Design review of the part built by this model. Coordinates are the model's own, in mm. A direction names the side the tool comes from. Round coordinates to 2 decimals unless told otherwise and drop trailing zeros. Order: outer loops, then holes, each group sorted by start corner. A loop starts at its lowest first (then second) coordinate and runs counter-clockwise, first axis right, second up. Notation, with made-up numbers: M 1.5,26 L 51.5,26 A26 ccw 51.5,48 Z; hole C 47.25,77.5 d5. An arc over 180 degrees is marked long. Write item = value, one per line. Start each with the question number.
```python
from build123d import *

# Parameters (mm, degrees)
SKETCH1_R           = 3.45
BOSS_EXTRUDE1_DEPTH = 2
BOSS_EXTRUDE2_START = 8.75
BOSS_EXTRUDE2_DEPTH = 8.75
CIRPATTERN1_COUNT   = 4


with BuildPart() as part:
    # Sketch1 → Boss-Extrude1 (new body)
    with BuildSketch(Plane(origin=(0, 0, 0), x_dir=(1, 0, 0), z_dir=(0, 1, 0))):
        with BuildLine():
            ThreePointArc((28.363609444, -42.985528487), (38.899494937, -38.899494937), (42.985528487, -28.363609444))
            ThreePointArc((42.985528487, -28.363609444), (51.5, 0), (42.985528487, 28.363609444))
            ThreePointArc((42.985528487, 28.363609444), (38.899494937, 38.899494937), (28.363609444, 42.985528487))
            ThreePointArc((28.363609444, 42.985528487), (0, 51.5), (-28.363609444, 42.985528487))
            ThreePointArc((-28.363609444, 42.985528487), (-38.899494937, 38.899494937), (-42.985528487, 28.363609444))
            ThreePointArc((-42.985528487, 28.363609444), (-51.5, 0), (-42.985528487, -28.363609444))
            ThreePointArc((-42.985528487, -28.363609444), (-38.899494937, -38.899494937), (-28.363609444, -42.985528487))
            ThreePointArc((-28.363609444, -42.985528487), (0, -51.5), (28.363609444, -42.985528487))
        make_face()
        with Locations(Location((14.5, 14.5, 0), (0, 0, 270))):
            Circle(SKETCH1_R, mode=Mode.SUBTRACT)
        with Locations(Location((-14.5, 14.5, 0), (0, 0, 270))):
            Circle(SKETCH1_R, mode=Mode.SUBTRACT)
        with Locations(Location((-14.5, -14.5, 0), (0, 0, 270))):
            Circle(SKETCH1_R, mode=Mode.SUBTRACT)
        with Locations(Location((14.5, -14.5, 0), (0, 0, 270))):
            Circle(SKETCH1_R, mode=Mode.SUBTRACT)
    extrude(amount=BOSS_EXTRUDE1_DEPTH)

    # Sketch2 → Boss-Extrude2 (add)
    with BuildSketch(Plane.XZ.offset(BOSS_EXTRUDE2_START)):
        with BuildLine():
            Line((43.690302721, -24.313729622), (45.001011803, -25.043141511))
            ThreePointArc((45.001011803, -25.043141511), (51.499991825, 0.029017326), (44.972762458, 25.093836632))
            Line((44.972762458, 25.093836632), (43.690302721, 24.313729622))
            ThreePointArc((43.690302721, 24.313729622), (50, 0), (43.690302721, -24.313729622))
        make_face()
    boss_extrude2 = extrude(amount=-BOSS_EXTRUDE2_DEPTH)

    # CirPattern1: Boss-Extrude2 ×4 about axis
    cirpattern1_axis = Axis((0, 0, 0), (0, 1, 0))
    for i in range(1, CIRPATTERN1_COUNT):
        add(boss_extrude2.rotate(cirpattern1_axis, i * 360 / CIRPATTERN1_COUNT))


solid = part.part
```
(1) Consider section A-A, the plane y = -5.25. Write out the cut boundary in (x, z).
(2) Consider section C-C, the plane x = 0. Write out the cut boundary in (y, z).
(3) For line 1 along X through (y, z) = (0.6, 14.5); line 2 along Y through (x, z) = (-22.5, 39); line 3 along Z through (x, y) = (6, -0.75), list the stretches that pass through material, from the lowest coordinate up. Write a range as [from, to].
(4) Consider section D-D, the plane x = -14.5. Write out the cut boundary in (y, z), then the cut area to 3 significant figures.
(5) Consider section B-B, the plane z = 14.5. Write out the cut boundary in (x, y), then the cut area to 3 significant figures.
(6) For faces 3 (the face through (0, -4, 50)), 4 (the face through (-1, 2, -1)), list the 3-axis set-ups (+Z, -Z, +X, -X, +Y, -Y) from which the entire face can be reached by the end or side of a thin tool; tool diameter is ignored.
(7) Insertion check: pin 1 (1 mm diameter, centred on x = 0.5, z = 5, fed in from -Y); pin 2 (1.5 mm diameter, centred on x = 3, y = -1.5, fed in from -Z); pin 3 (6 mm diameter, centred on y = -2.5, z = -16, fed in from -X). Each pin has a flat end and moves straight along its axis. Give the tip position at first contact, or say it passes through.
(8) Draft analysis for pull direction Z (two halves, no side actions). For faces 1 (the face through (-0.1, -8.75, 50.2)), 2 (the face through (-11.08, 0.99, 14.05)), state which applies: pulls with the +Z half, pulls with the -Z half, needs draft (parallel to the pull), parting line crosses it, or undercut.
Completed:
q1.outline = M -45,25.04 A51.5 ccw -44.97,-25.09 L -43.69,-24.31 A50 cw -43.69,24.31 Z; M -25.09,44.97 L -24.31,43.69 A50 cw 24.31,43.69 L 25.04,45 A51.5 ccw Z; M -25.04,-45 A51.5 ccw 25.09,-44.97 L 24.31,-43.69 A50 cw -24.31,-43.69 Z; M 43.69,-24.31 L 45,-25.04 A51.5 ccw 44.97,25.09 L 43.69,24.31 A50 cw Z
q2.outline = M -8.75,-51.5 L 2,-51.5 L 2,51.5 L -8.75,51.5 L -8.75,50 L 0,50 L 0,-50 L -8.75,-50 Z
q3.line_1 = [-49.42, -17.95], [-11.05, 11.05], [17.95, 49.42]
q3.line_2 = [0, 2]
q3.line_3 = [-51.15, -49.64], [49.64, 51.15]
q4.outline = M -8.75,-49.42 L 2,-49.42 L 2,-17.95 L 0,-17.95 L 0,-47.85 L -8.75,-47.85 Z; M -8.75,47.85 L 0,47.85 L 0,17.95 L 2,17.95 L 2,49.42 L -8.75,49.42 Z; M 0,-11.05 L 2,-11.05 L 2,11.05 L 0,11.05 Z
q4.area = 197 mm2
q5.outline = M -49.42,-8.75 L -47.85,-8.75 L -47.85,0 L -17.95,0 L -17.95,2 L -49.42,2 Z; M -11.05,0 L 11.05,0 L 11.05,2 L -11.05,2 Z; M 17.95,0 L 47.85,0 L 47.85,-8.75 L 49.42,-8.75 L 49.42,2 L 17.95,2 Z
q5.area = 197 mm2
q6.face_3 = -Y
q6.face_4 = +Z, -Z, +X, -X, +Y
q7.pin_1 = 0
q7.pin_2 = -51.45
q7.pin_3 = -49.83
q8.face_1 = needs draft
q8.face_2 = undercut
